For this review, take the finished solid that the model builds, in its own axes (mm). A direction names the side the tool comes from. Coordinates: 2 decimals unless noted, no trailing zeros. Loops run counter-clockwise (first coordinate to the right, second up) from the corner with the lowest first, then second, coordinate; pieces in that order, holes last. Notation, with made-up numbers: M -16,47 L 15,47 A27 ccw 15,73 Z; hole C 49.25,56 d7. An arc over 180 degrees is marked long. Write item = value, one per line.
from build123d import *

# Parameters (mm, degrees)
BOSS_EXTRUDE1_DEPTH  = 1.5625
MIRROR4_COPY_1_DEPTH = 1.5625
FILLET1_R            = 5


with BuildPart() as part:
    # Sketch1 → Boss-Extrude1 (new body, symmetric)
    with BuildSketch(Plane(origin=(0, 0, 0), x_dir=(1, 0, 0), z_dir=(0, 1, 0))):
        Polygon((0, 33.5), (35, 33.5), (35, 24), (28.5, 24), (28.5, 26), (26, 26), (26, 24), (24, 24), (24, 21), (26, 21), (26, 19), (28.5, 19), (28.5, 21), (35, 21), (35, 0), (0, 0), align=None)
    boss_extrude1 = extrude(amount=BOSS_EXTRUDE1_DEPTH, both=True)

    # Mirror1: Boss-Extrude1 across plane
    add(boss_extrude1.mirror(Plane(origin=(0, 0, 0), x_dir=(0, 0, 1), z_dir=(1, 0, 0))))

    # Mirror4: Boss-Extrude1 across plane
    add(boss_extrude1.mirror(Plane.XY))

    # Mirror4 copy 1 sketch → Mirror4 copy 1 (add, symmetric)
    with BuildSketch(Plane(origin=(0, 0, 0), x_dir=(-1, 0, 0), z_dir=(0, 1, 0))):
        Polygon((0, 33.5), (35, 33.5), (35, 24), (28.5, 24), (28.5, 26), (26, 26), (26, 24), (24, 24), (24, 21), (26, 21), (26, 19), (28.5, 19), (28.5, 21), (35, 21), (35, 0), (0, 0), align=None)
    extrude(amount=MIRROR4_COPY_1_DEPTH, both=True)

    # Fillet1
    fillet1_edges = [part.edges().sort_by_distance(p)[0] for p in [
        (35, 0, 33.5),
        (35, 0, -33.5),
        (-35, 0, -33.5),
        (-35, 0, 33.5),
    ]]
    fillet(fillet1_edges, radius=FILLET1_R)


solid = part.part
Q1. Machinability: for faces 4 (the face through (32, 0, -24)), 5 (the face through (-35, 0, 0)), 6 (the face through (-32, 0, -24)), 7 (the face through (0, 0, 33.5)), 8 (the face through (-28.5, 0, -25)), which of the approach directions +Z, -Z, +X, -X, +Y, -Y give a long, thin tool a straight path to every point of the face, cutting with its end or side? Answer none if there is none.
Solved:
face_4 = +X, +Y, -Y
face_5 = +Z, -Z, -X, +Y, -Y
face_6 = -X, +Y, -Y
face_7 = +Z, +X, -X, +Y, -Y
face_8 = +Y, -Y
Q2. For line 1 along Z through (x, y) = (-30, 0.8); line 2 along Z through (x, y) = (-27, -0.1), list the stretches that pass through material, from the lowest coordinate up.
Solved:
line_1 = -33.5 to -24, -21 to 21, 24 to 33.5
line_2 = -33.5 to -26, -19 to 19, 26 to 33.5
Q3. Add section A-A (x = 25). Write out the cut boundary in (y, z), and give its area (3 significant figures).
Solved:
outline = M -1.56,-33.5 L 1.56,-33.5 L 1.56,-24 L -1.56,-24 Z; M -1.56,-21 L 1.56,-21 L 1.56,21 L -1.56,21 Z; M -1.56,24 L 1.56,24 L 1.56,33.5 L -1.56,33.5 Z
area = 191 mm²
Q4. For pin 1 Ø0.9 at (x, y) = (-31, 0) entering from +Z; pin 2 Ø1.5 at (y, z) = (0, -23) entering from +X; pin 3 Ø1.5 at (y, z) = (0, 22) entering from -X, all flat-tipped, find the tip position at first contact; note any pin that passes through.
Solved:
pin_1 = 33.47
pin_2 = 24
pin_3 = -24
Q5. Draft analysis for pull direction Z (two halves, no side actions). For faces 1 (the face through (-35, 0, -26)), 2 (the face through (-33.5, -0.02, 32.07)), 3 (the face through (32, 0, 24)), state which applies: +Z half, -Z half, draft (parallel to the pull), parting line (faces both ways), or undercut.
Solved:
face_1 = draft
face_2 = +Z half
face_3 = undercut
